Geometry check sheet. Reference: the model listing, model coordinates, mm. A direction names the side the tool comes from. Round coordinates to 2 decimals unless told otherwise and drop trailing zeros. Write each loop counter-clockwise with the first axis right and the second up, starting at its lowest first coordinate (ties: lowest second). Pieces come first, ordered by that corner, then holes. Notation, with made-up numbers: (-36, -37) - (-24, -37) arc R22 cw to (-24, -2) - close; hole circle Ø1 at (-7.5, -30). An arc over 180 degrees is marked (long way). Return JSON: item names as keys, results as strings.
Autodesk Inventor part; units mm, degrees
ref_plane "YZ Plane" through (0, 0, 0) normal (1, 0, 0) x (0, 1, 0)
ref_plane "XZ Plane" through (0, 0, 0) normal (0, 1, 0) x (-1, 0, 0)
ref_plane "XY Plane" through (0, 0, 0) normal (0, 0, 1) x (1, 0, 0)
sketch "Sketch1" plane through (0, 0, 0) normal (0, 0, 1) x (1, 0, 0)
  line L0 (-9.8382, 8.8164) -> (64.1618, 8.8164)
  line L1 (66.1618, 6.8164) -> (66.1618, -53.1836)
  line L2 (64.1618, -55.1836) -> (-9.8382, -55.1836)
  line L3 (-11.8382, -53.1836) -> (-11.8382, 6.8164)
  line L4 (-9.8382, 8.8164) -> (-11.8382, 6.8164)
  line L5 (64.1618, 8.8164) -> (66.1618, 6.8164)
  line L6 (66.1618, -53.1836) -> (64.1618, -55.1836)
  line L7 (-11.8382, -53.1836) -> (-9.8382, -55.1836)
  circle A0 centre (9.1618, 5.8164) radius 1.25
  circle A1 centre (9.1618, -52.1836) radius 1.25
  circle A2 centre (-7.8382, 4.8164) radius 1.75
  circle A3 centre (-7.8382, -51.1836) radius 1.75
  circle A4 centre (62.1618, -51.1836) radius 1.75
  circle A5 centre (62.1618, 4.8164) radius 1.75
  point P0 (0, 0)
  point P1 (-11.8382, 8.8164)
  point P2 (66.1618, -55.1836)
  point P3 (66.1618, 8.8164)
  point P4 (-11.8382, -55.1836)
  dimension "d0" = 78
  dimension "d1" = 64
  dimension "d2" = 2
  dimension "d3" = 2
  dimension "d4" = 2
  dimension "d5" = 2
  dimension "d6" = 2
  dimension "d7" = 2
  dimension "d8" = 2
  dimension "d9" = 2
  dimension "d10" = 2.5
  dimension "d11" = 21
  dimension "d12" = 3
  dimension "d13" = 2.5
  dimension "d14" = 3
  dimension "d15" = 21
  dimension "d16" = 3.5
  dimension "d17" = 4
  dimension "d18" = 4
  dimension "d19" = 3.5
  dimension "d20" = 4
  dimension "d21" = 4
  dimension "d22" = 3.5
  dimension "d23" = 4
  dimension "d24" = 4
  dimension "d25" = 3.5
  dimension "d26" = 4
  dimension "d27" = 4
extrude "Extrusion1" add sketch "Sketch1" along normal blind 2
sketch "Sketch2" plane through (0, 0, 2) normal (0, 0, 1) x (1, 0, 0)
  line L0 (66.1618, -53.1836) -> (66.1618, 6.8164)
  line L1 (66.1618, 0.8164) -> (51.1618, 0.8164)
  line L2 (51.1618, 0.8164) -> (51.1618, -13.1836)
  line L3 (51.1618, -13.1836) -> (66.1618, -13.1836)
  line L4 (66.1618, -13.1836) -> (66.1618, 0.8164)
  line L5 (64.1618, 8.8164) -> (-9.8382, 8.8164)
  line L6 (66.1618, -47.1836) -> (51.1618, -47.1836)
  line L7 (51.1618, -47.1836) -> (51.1618, -33.1836)
  line L8 (51.1618, -33.1836) -> (66.1618, -33.1836)
  line L9 (66.1618, -33.1836) -> (66.1618, -47.1836)
  line L10 (-9.8382, -55.1836) -> (64.1618, -55.1836)
  point P0 (0, 0)
  dimension "d30" = 15
  dimension "d31" = 14
  dimension "d32" = 8
  dimension "d33" = 14
  dimension "d34" = 8
extrude "Extrusion2" add sketch "Sketch2" along normal blind 14
sketch "Sketch3" plane through (66.1618, -53.1836, 0) normal (1, 0, 0) x (0, 0, -1)
  circle A0 centre (-9, 13) radius 5.5
  line L0 (-2, 6) -> (-16, 6)
  line L1 (-16, 6) -> (-16, 20)
  circle A1 centre (-9, 47) radius 5.5
  line L2 (-16, 40) -> (-16, 54)
  line L3 (-2, 40) -> (-16, 40)
  point P0 (0, 53.1836)
  dimension "d37" = 11
  dimension "d38" = 7
  dimension "d39" = 7
  dimension "d40" = 11
  dimension "d41" = 7
  dimension "d42" = 7
extrude "Extrusion3" cut sketch "Sketch3" against normal up to surface (15 mm away)
chamfer "Chamfer1" distance 3 angle 45 4 edges at (58.6618, 0.8164, 16) (58.6618, -13.1836, 16) (58.6618, -33.1836, 16) (58.6618, -47.1836, 16)
properties part number "powersupplymount"
(1) Section check A-A, the plane z = 9. Enter the section's corners in (x, y).
Response values:
{"outline": "(51.16, -47.18) - (66.16, -47.18) - (66.16, -45.68) - (51.16, -45.68) - close; (51.16, -34.68) - (66.16, -34.68) - (66.16, -33.18) - (51.16, -33.18) - close; (51.16, -13.18) - (66.16, -13.18) - (66.16, -11.68) - (51.16, -11.68) - close; (51.16, -0.68) - (66.16, -0.68) - (66.16, 0.82) - (51.16, 0.82) - close"}
(2) Section check C-C, the plane x = 53. Enter the section's corners in (y, z), plus the area to 3 significant figures.
Response values:
{"outline": "(-55.18, 0) - (8.82, 0) - (8.82, 2) - (0.82, 2) - (0.82, 13) - (-2.18, 16) - (-10.18, 16) - (-13.18, 13) - (-13.18, 2) - (-33.18, 2) - (-33.18, 13) - (-36.18, 16) - (-44.18, 16) - (-47.18, 13) - (-47.18, 2) - (-55.18, 2) - close; hole circle Ø11 at (-40.18, 9); hole circle Ø11 at (-6.18, 9)", "area": "312 mm^2"}
(3) Section check D-D, the plane y = -31. Enter the section's corners in (x, z), plus the area to 3 significant figures.
Response values:
{"outline": "(-11.84, 0) - (66.16, 0) - (66.16, 2) - (-11.84, 2) - close", "area": "156 mm^2"}
(4) Material ranges on line 1 along Y through (x, z) = (58, 3); line 2 along Y through (x, z) = (54, 10.5); line 3 along Z through (x, y) = (-4.5, -25), recorded low to high. Write a range as [from, to].
Response values:
{"line 1": "y = [-47.18, -33.18], [-13.18, 0.82]", "line 2": "y = [-47.18, -45.48], [-34.89, -33.18], [-13.18, -11.48], [-0.89, 0.82]", "line 3": "z = [0, 2]"}
(5) Gauge pin test, flat ends, axial feed: pin 1 (8 mm diameter, centred on y = -42.5, z = 10, fed in from +X); pin 2 (5.5 mm diameter, centred on x = 61, z = 10, fed in from +Y); pin 3 (2 mm diameter, centred on x = 62.16, y = 4.82, fed in from -Z); pin 4 (5.5 mm diameter, centred on x = 56.5, z = 9.5, fed in from -Y). Record the tip position at first contact, or that the pin passes through.
Response values:
{"pin 1": "stops at x = 66.16", "pin 2": "stops at y = 0.82", "pin 3": "passes through", "pin 4": "stops at y = -47.18"}
(6) Release check for a two-part mould opening along Y. For faces 1 (the face through (59, -6, 16)), 2 (the face through (28, -55.184, 1)), 3 (the face through (58.77, -8.29, 3.92)) record: pulls with the +Y half, pulls with the -Y half, needs draft (parallel to the pull), parting line crosses it, or undercut.
Response values:
{"face 1": "needs draft", "face 2": "pulls with the -Y half", "face 3": "undercut"}
(7) Access from +Z, -Z, +X, -X, +Y, -Y to the whole of each face (thin tool, end or side, straight path). Record for faces 4 (the face through (60.77, 5.88, 0.99)), 5 (the face through (-10.85, -54.17, 0.99)), 6 (the face through (51.162, -43, 4)), 7 (the face through (59, -33.184, 7)), 8 (the face through (59, -47.184, 7)).
Response values:
{"face 4": "+Z, -Z", "face 5": "+Z, -Z, -X, -Y", "face 6": "+Z, -X, +Y, -Y", "face 7": "+Z, +X, -X", "face 8": "+Z, +X, -X, -Y"}
(8) Section check B-B, the plane y = -42.5. Enter the section's corners in (x, z), plus the area to 3 significant figures.
Response values:
{"outline": "(-11.84, 0) - (66.16, 0) - (66.16, 4.01) - (51.16, 4.01) - (51.16, 2) - (-11.84, 2) - close; (51.16, 13.99) - (66.16, 13.99) - (66.16, 16) - (51.16, 16) - close", "area": "216 mm^2"}
